Source: three-view drawing plus pictorial views. Frame: mm from the lowest corner of the part. A direction names the side the tool comes from. Give positions to 0.01 mm unless a question says otherwise; leave off trailing zeros. Loops run counter-clockwise (first coordinate to the right, second up) from the corner with the lowest first, then second, coordinate; pieces in that order, holes last.
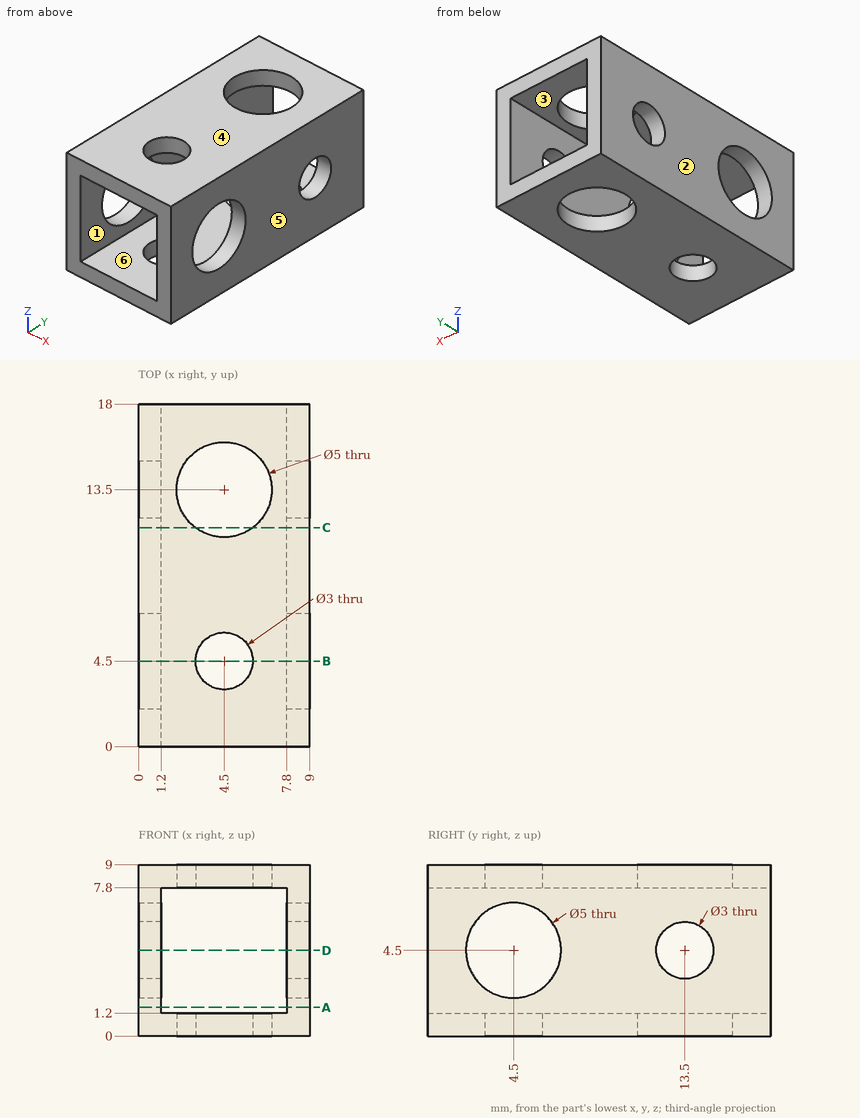
1) Cut plane D-D (z = 4.5). Return loops of the section in (x, y).
Checks:
outline: (0, 0) - (1.2, 0) - (1.2, 2) - (0, 2) - close; (0, 7) - (1.2, 7) - (1.2, 12) - (0, 12) - close; (0, 15) - (1.2, 15) - (1.2, 18) - (0, 18) - close; (7.8, 0) - (9, 0) - (9, 2) - (7.8, 2) - close; (7.8, 7) - (9, 7) - (9, 12) - (7.8, 12) - close; (7.8, 15) - (9, 15) - (9, 18) - (7.8, 18) - close
2) Pull-direction query (X, two-part tool) for the marked faces 3, 4, 5 and 6; classes: released by +X, released by -X, zero draft, split by the parting line, or undercut.
Checks:
face 3: undercut
face 4: zero draft
face 5: released by +X
face 6: undercut
3) Cut plane B-B (y = 4.5). Return loops of the section in (x, z).
Checks:
outline: (0, 0) - (3, 0) - (3, 1.2) - (1.2, 1.2) - (1.2, 2) - (0, 2) - close; (0, 7) - (1.2, 7) - (1.2, 7.8) - (3, 7.8) - (3, 9) - (0, 9) - close; (6, 0) - (9, 0) - (9, 2) - (7.8, 2) - (7.8, 1.2) - (6, 1.2) - close; (6, 7.8) - (7.8, 7.8) - (7.8, 7) - (9, 7) - (9, 9) - (6, 9) - close
4) Cut plane C-C (y = 11.5). Return loops of the section in (x, z), and give its area (3 significant figures).
Checks:
outline: (0, 0) - (3, 0) - (3, 1.2) - (1.2, 1.2) - (1.2, 7.8) - (3, 7.8) - (3, 9) - (0, 9) - close; (6, 0) - (9, 0) - (9, 9) - (6, 9) - (6, 7.8) - (7.8, 7.8) - (7.8, 1.2) - (6, 1.2) - close
area: 30.2 mm2
5) Reachability of the marked faces 1 and 2 from +Z, -Z, +X, -X, +Y, -Y: full face, straight path, thin tool, end or side. Return the list, or none.
Checks:
face 1: +Y, -Y
face 2: +Z, -Z, -X, +Y, -Y
6) Ray query, probe 1 along Y at (x, z) = (4.5, 8.6); probe 2 along Y at (x, z) = (0.85, 4.5); probe 3 along X at (y, z) = (11.5, 7.25). Return the intervals inside material, ascending.
Checks:
probe 1: y = 0 to 3, 6 to 11, 16 to 18
probe 2: y = 0 to 2, 7 to 12, 15 to 18
probe 3: x = 0 to 1.2, 7.8 to 9
7) Cut plane A-A (z = 1.5). Return loops of the section in (x, y), and give its area (3 significant figures).
Checks:
outline: (0, 0) - (1.2, 0) - (1.2, 18) - (0, 18) - close; (7.8, 0) - (9, 0) - (9, 18) - (7.8, 18) - close
area: 43.2 mm2
